Source: CAD feature listing. Evaluate the final solid. Frame: model axes, mm. Coordinates: 2 decimals unless noted, no trailing zeros. Order: outer loops, then holes, each group sorted by start corner. A loop starts at its lowest first (then second) coordinate and runs counter-clockwise, first axis right, second up. Notation, with made-up numbers: (-26.75, -36.75) -> (-3.75, -36.75) arc R13 cw to (-3.75, -21.75) -> close; hole circle Ø2 at (0, 18.5). An arc over 180 degrees is marked (long way). Put each result on its own line as item: value.
from build123d import *

# Parameters (mm, degrees)
F0_R     = 15
F1_DEPTH = 5
F2_DEPTH = 10


with BuildPart() as f1:
    # F0 (on Front) → F1 (new body)
    with BuildSketch(Plane.XZ):
        with BuildLine():
            ThreePointArc((22.882668, 119.834872), (24.464941, 124.759235), (25, 129.903811))
            ThreePointArc((25, 129.903811), (-5.144575, 154.368752), (-22.882668, 119.834872))
            ThreePointArc((-22.882668, 119.834872), (0, 104.903811), (22.882668, 119.834872))
        make_face()
        with Locations((0, 129.903811)):
            Circle(F0_R, mode=Mode.SUBTRACT)
        with BuildLine():
            ThreePointArc((22.882668, 119.834872), (0, 104.903811), (-22.882668, 119.834872))
            ThreePointArc((-22.882668, 119.834872), (-26.233796, 58.447359), (-77.721377, 24.851441))
            ThreePointArc((-77.721377, 24.851441), (-58.312197, 18.614973), (-50, 0))
            ThreePointArc((-50, 0), (-51.240452, -7.777138), (-54.83871, -14.782502))
            ThreePointArc((-54.83871, -14.782502), (0, 13.009092), (54.83871, -14.782502))
            ThreePointArc((54.83871, -14.782502), (53.349365, 12.5), (77.721377, 24.851441))
            ThreePointArc((77.721377, 24.851441), (26.233796, 58.447359), (22.882668, 119.834872))
        make_face()
        with BuildLine():
            ThreePointArc((-50, 0), (-58.312197, 18.614973), (-77.721377, 24.851441))
            ThreePointArc((-77.721377, 24.851441), (-96.650635, -12.5), (-54.83871, -14.782502))
            ThreePointArc((-54.83871, -14.782502), (-51.240452, -7.777138), (-50, 0))
        make_face()
        with Locations((-75, 0)):
            Circle(F0_R, mode=Mode.SUBTRACT)
        with BuildLine():
            ThreePointArc((100, 0), (93.614973, 16.687803), (77.721377, 24.851441))
            ThreePointArc((77.721377, 24.851441), (53.349365, 12.5), (54.83871, -14.782502))
            ThreePointArc((54.83871, -14.782502), (82.777138, -23.759548), (100, 0))
        make_face()
        with Locations((75, 0)):
            Circle(F0_R, mode=Mode.SUBTRACT)
    extrude(amount=F1_DEPTH)

    # F0 (on Front) → F2 (join)
    with BuildSketch(Plane.XZ):
        with BuildLine():
            ThreePointArc((22.882668, 119.834872), (24.464941, 124.759235), (25, 129.903811))
            ThreePointArc((25, 129.903811), (-5.144575, 154.368752), (-22.882668, 119.834872))
            ThreePointArc((-22.882668, 119.834872), (0, 104.903811), (22.882668, 119.834872))
        make_face()
        with Locations((0, 129.903811)):
            Circle(F0_R, mode=Mode.SUBTRACT)
        with BuildLine():
            ThreePointArc((22.882668, 119.834872), (0, 104.903811), (-22.882668, 119.834872))
            ThreePointArc((-22.882668, 119.834872), (-26.233796, 58.447359), (-77.721377, 24.851441))
            ThreePointArc((-77.721377, 24.851441), (-58.312197, 18.614973), (-50, 0))
            ThreePointArc((-50, 0), (-51.240452, -7.777138), (-54.83871, -14.782502))
            ThreePointArc((-54.83871, -14.782502), (0, 13.009092), (54.83871, -14.782502))
            ThreePointArc((54.83871, -14.782502), (53.349365, 12.5), (77.721377, 24.851441))
            ThreePointArc((77.721377, 24.851441), (26.233796, 58.447359), (22.882668, 119.834872))
        make_face()
        with BuildLine():
            ThreePointArc((-50, 0), (-58.312197, 18.614973), (-77.721377, 24.851441))
            ThreePointArc((-77.721377, 24.851441), (-96.650635, -12.5), (-54.83871, -14.782502))
            ThreePointArc((-54.83871, -14.782502), (-51.240452, -7.777138), (-50, 0))
        make_face()
        with Locations((-75, 0)):
            Circle(F0_R, mode=Mode.SUBTRACT)
        with BuildLine():
            ThreePointArc((100, 0), (93.614973, 16.687803), (77.721377, 24.851441))
            ThreePointArc((77.721377, 24.851441), (53.349365, 12.5), (54.83871, -14.782502))
            ThreePointArc((54.83871, -14.782502), (82.777138, -23.759548), (100, 0))
        make_face()
        with Locations((75, 0)):
            Circle(F0_R, mode=Mode.SUBTRACT)
    extrude(amount=F2_DEPTH)


solid = f1.part
1. Cut plane C-C on z = 139. Output: boundary loops of the cut face in (x, y).
Numbers:
outline: (-23.29, -10) -> (-11.93, -10) -> (-11.93, 0) -> (-23.29, 0) -> close; (11.93, -10) -> (23.29, -10) -> (23.29, 0) -> (11.93, 0) -> close
2. Cut plane D-D on x = 30. Output: boundary loops of the cut face in (y, z), plus the area to 3 significant figures.
Numbers:
outline: (-10, 6.03) -> (0, 6.03) -> (0, 52.63) -> (-10, 52.63) -> close
area: 466 mm2
3. Pull-direction query (X, two-part tool) for faces 1 (the cylindrical face through (-1, -5, 13)), 2 (the cylindrical face through (-25.792, -4.93, 59.224)), 3 (the cylindrical face through (24.45, -4.93, 124.69)), 4 (the flat face through (0, 0, 45)); classes: pulls with the +X half, pulls with the -X half, needs draft (parallel to the pull), parting line crosses it, or undercut.
Numbers:
face 1: undercut
face 2: pulls with the -X half
face 3: pulls with the +X half
face 4: needs draft
4. Ray query, line 1 along Z through (x, y) = (0, -3); line 2 along Z through (x, y) = (75, -3.75); line 3 along X through (y, z) = (-5, -6.5). Return the intervals inside material, ascending.
Numbers:
line 1: z = 13.01 to 114.9, 144.9 to 154.9
line 2: z = -25 to -15, 15 to 25.21
line 3: x = -99.14 to -88.52, -61.48 to -47.67, 47.67 to 61.48, 88.52 to 99.14
5. Cut plane A-A on x = 0. Output: boundary loops of the cut face in (y, z).
Numbers:
outline: (-10, 13.01) -> (0, 13.01) -> (0, 114.9) -> (-10, 114.9) -> close; (-10, 144.9) -> (0, 144.9) -> (0, 154.9) -> (-10, 154.9) -> close
6. Cut plane B-B on y = -7.5. Output: boundary loops of the cut face in (x, z).
Numbers:
outline: (-77.72, 24.85) arc R25 ccw (long way) to (-54.84, -14.78) arc R68 cw to (54.84, -14.78) arc R25 ccw to (100, 0) arc R25 ccw to (77.72, 24.85) arc R68 cw to (22.88, 119.83) arc R25 ccw to (25, 129.9) arc R25 ccw (long way) to (-22.88, 119.83) arc R68 cw to start; hole circle Ø30 at (-75, 0); hole circle Ø30 at (0, 129.9); hole circle Ø30 at (75, 0)
7. First-contact query: pin 1 (2 mm diameter, centred on x = -61, y = -8.5, fed in from -Z); pin 2 (1.5 mm diameter, centred on x = -62.5, y = -5, fed in from +Z); pin 3 (10 mm diameter, centred on x = -10, z = 100.5, fed in from +Y); pin 4 (5 mm diameter, centred on y = -4.5, z = 87, fed in from +X). Flat tips, straight axial feed; report the tip coordinate or a pass-through.
Numbers:
pin 1: stops at z = -21.35
pin 2: stops at z = 28.59
pin 3: stops at y = 0
pin 4: stops at x = 17.59
